Build history of the part. All positions in model axes, mm. Round coordinates to 2 decimals unless told otherwise and drop trailing zeros. Order: outer loops, then holes, each group sorted by start corner. A loop starts at its lowest first (then second) coordinate and runs counter-clockwise, first axis right, second up. Notation, with made-up numbers: (-36, 21) -> (-16, 21) arc R23 ccw to (-16, 49) -> close; hole circle Ø10 at (21, -25). An arc over 180 degrees is marked (long way). Answer as a JSON object with one key per item and string values.
from build123d import *

# Parameters (mm, degrees)
BOSS_EXTRUDE1_DEPTH      = 950
BOSS_EXTRUDE1_DEPTH_BACK = 286
SKETCH1_R                = 9.313662058
BOSS_EXTRUDE2_DEPTH      = 3
BOSS_EXTRUDE2_DEPTH_BACK = 5
BOSS_EXTRUDE2_START      = -5


with BuildPart() as part:
    # Sketch1 → Boss-Extrude1 (new, two sides: drawn at the far end of the back side and taken through both)
    with BuildSketch(Plane(origin=(0, 4239.077255807, 0), x_dir=(1, 0, 0), z_dir=(0, 1, 0)).offset(-BOSS_EXTRUDE1_DEPTH_BACK)):
        with Locations(Location((838.898443774, -1523.820122511, 0), (0, 0, 270))):
            Circle(SKETCH1_R)
    extrude(amount=BOSS_EXTRUDE1_DEPTH + BOSS_EXTRUDE1_DEPTH_BACK)

    # Sketch2 → Boss-Extrude2 (add, two sides: drawn at the far end of the back side and taken through both)
    with BuildSketch(Plane(origin=(0, 5189.077255807, 0), x_dir=(1, 0, 0), z_dir=(0, 1, 0)).offset(BOSS_EXTRUDE2_START - BOSS_EXTRUDE2_DEPTH_BACK)):
        with BuildLine():
            Line((829.584781716, -1561.145044768), (829.584781716, -1523.820122511))
            Line((829.584781716, -1523.820122511), (848.212105832, -1523.820122511))
            ThreePointArc((848.212105832, -1523.820122511), (846.628688281, -1546.340428779), (829.584781716, -1561.145044768))
        make_face()
    extrude(amount=BOSS_EXTRUDE2_DEPTH + BOSS_EXTRUDE2_DEPTH_BACK)


solid = part.part
1) Cut at A-A, the plane x = 844.5. Give the cut face in (y, z), plus the area to 3 significant figures.
Checked values:
{"outline": "(3953.08, 1516.38) -> (5189.08, 1516.38) -> (5189.08, 1531.26) -> (5187.08, 1531.26) -> (5187.08, 1549.94) -> (5179.08, 1549.94) -> (5179.08, 1531.26) -> (3953.08, 1531.26) -> close", "area": "18,500 mm²"}
2) Cut at C-C, the plane y = 4616. Give the cut face in (x, z), plus the area to 3 significant figures.
Checked values:
{"outline": "circle Ø18.63 at (838.9, 1523.82)", "area": "273 mm²"}
3) Flat gauge pins, fed straight in: pin 1 Ø4 at (x, z) = (840.5, 1544.5) entering from +Y; pin 2 Ø8 at (x, y) = (834.5, 4317.5) entering from +Z; pin 3 Ø4 at (x, y) = (835.5, 4123.5) entering from -Z. Where does each tip first touch, or does it go through?
Checked values:
{"pin 1": "stops at y = 5187.08", "pin 2": "stops at z = 1533.13", "pin 3": "stops at z = 1514.61"}
4) Cut at B-B, the plane z = 1540.5. Give the cut face in (x, y), plus the area to 3 significant figures.
Checked values:
{"outline": "(829.58, 5179.08) -> (848.81, 5179.08) -> (848.81, 5187.08) -> (829.58, 5187.08) -> close", "area": "154 mm²"}
5) Probe L1, parallel to Y at x = 843.75, z = 1535; L2, parallel to X at y = 4894, z = 1522; L3, parallel to Z at x = 841, y = 4318. List the from-to ranges inside material, lowest first. Write a range as from..to.
Checked values:
{"L1": "y = 5179.08..5187.08", "L2": "x = 829.76..848.03", "L3": "z = 1514.75..1532.89"}
